Part model, mm, in its own coordinate system. A direction names the side the tool comes from. Coordinates: 2 decimals unless noted, no trailing zeros. Order: outer loops, then holes, each group sorted by start corner. A loop starts at its lowest first (then second) coordinate and runs counter-clockwise, first axis right, second up. Notation, with made-up numbers: M 9,82 L 68,82 A11 ccw 68,101 Z; hole C 61.25,-25 d6. An arc over 180 degrees is marked long. Answer in a Markdown table with one row per item. Add a question column.
from build123d import *

# Parameters (mm, degrees)
BOSS_EXTRUDE1_DEPTH = 10
BOSS_EXTRUDE2_DEPTH = 8
SKETCH4_R           = 13
CUT_EXTRUDE2_DEPTH  = 77.40353395
SKETCH5_W           = 4
SKETCH5_H           = 38
SKETCH5_R           = 1
BOSS_EXTRUDE3_DEPTH = 10


with BuildPart() as part:
    # Sketch1 → Boss-Extrude1 (new body)
    with BuildSketch(Plane(origin=(0, 0, 0), x_dir=(0, 1, 0), z_dir=(0, 0, 1))):
        with BuildLine():
            Line((-25, -37.5), (25, -37.5))
            ThreePointArc((25, -37.5), (33.838834765, -33.838834765), (37.5, -25))
            Line((37.5, -25), (37.5, 25))
            ThreePointArc((37.5, 25), (33.838834765, 33.838834765), (25, 37.5))
            Line((25, 37.5), (-25, 37.5))
            ThreePointArc((-25, 37.5), (-33.838834765, 33.838834765), (-37.5, 25))
            Line((-37.5, 25), (-37.5, -25))
            ThreePointArc((-37.5, -25), (-33.838834765, -33.838834765), (-25, -37.5))
        make_face()
    extrude(amount=BOSS_EXTRUDE1_DEPTH)

    # Sketch2 → Boss-Extrude2 (add)
    with BuildSketch(Plane.YZ.offset(37.5)):
        with BuildLine():
            ThreePointArc((14.587782351, 53.492363969), (0, 65), (-14.587782351, 53.492363969))
            Line((-14.587782351, 53.492363969), (-25, 10))
            Line((-25, 10), (25, 10))
            Line((25, 10), (14.587782351, 53.492363969))
        make_face()
        with BuildLine():
            ThreePointArc((0, 44), (-5.795554958, 48.447085729), (-3, 55.196152423))
            Line((-3, 55.196152423), (3, 55.196152423))
            ThreePointArc((3, 55.196152423), (5.795554958, 48.447085729), (0, 44))
        make_face(mode=Mode.SUBTRACT)
    boss_extrude2 = extrude(amount=-BOSS_EXTRUDE2_DEPTH)

    # Mirror1: Boss-Extrude2 across plane
    add(boss_extrude2.mirror(Plane(origin=(0, 0, 0), x_dir=(0, 0, 1), z_dir=(1, 0, 0))))

    # Sketch4 → Cut-Extrude2 (cut, through all)
    with BuildSketch(Plane.XY.offset(10)):
        Circle(SKETCH4_R)
    extrude(amount=-CUT_EXTRUDE2_DEPTH, mode=Mode.SUBTRACT)

    # Sketch5 → Boss-Extrude3 (add)
    # profile 1 of 2: a face of its own
    with BuildSketch(Plane.XY.offset(10)):
        with Locations((-15, 12.5)):
            Rectangle(SKETCH5_W, SKETCH5_H)
        with Locations((-15, -4.5)):
            Circle(SKETCH5_R, mode=Mode.SUBTRACT)
        with Locations((-15, 29.5)):
            Circle(SKETCH5_R, mode=Mode.SUBTRACT)
    # profile 2 of 2: a face of its own
    with BuildSketch(Plane.XY.offset(10)):
        with Locations((15, 12.5)):
            Rectangle(SKETCH5_W, SKETCH5_H)
        with Locations((15, -4.5)):
            Circle(SKETCH5_R, mode=Mode.SUBTRACT)
        with Locations((15, 29.5)):
            Circle(SKETCH5_R, mode=Mode.SUBTRACT)
    extrude(amount=BOSS_EXTRUDE3_DEPTH)


solid = part.part
(1) Drop flat-ended pins along their axis: P1, Ø1.6, axis at x = 15, y = 29.5, coming from the +Z side; P2, Ø4.5, axis at x = -16, z = 16.5, coming from the -Y side; P3, Ø2, axis at x = -15.5, z = 16.5, coming from the +Y side. Give the stop position or say it passes through.
(2) Slice it at D-D (y = -21.5). List the corners of the cut face in (x, z).
(3) 3-axis set-ups, long thin cutter, end or side, ignore diameter. For faces 4 (the cylindrical face through (-10.316, -7.91, 5.07)), 5 (the flat face through (-15, -6.5, 15)), 6 (the cylindrical face through (15.54, 30.34, 14.93)), 7 (the flat face through (15, 31.5, 15)), 8 (the flat face through (13, 12, 15)): which of +Z, -Z, +X, -X, +Y, -Y reach the whole face in a straight line?
(4) Pull direction Y, two halves, no side cores. Call faces 1 (the cylindrical face through (-33.935, -33.741, 4.93)), 2 (the cylindrical face through (-34, 0, 65)), 3 (the flat face through (-15, -5, 10)): pulls with the +Y half, pulls with the -Y half, needs draft (parallel to the pull), parting line crosses it, or undercut.
(5) Slice it at A-A (x = 12). List the corners of the cut face in (y, z).
(6) Wall check: line 1 (Y direction, x = -15, z = 13); line 2 (X direction, y = -11, z = 10.5); line 3 (X direction, y = -4, z = 15). Give the ranges that are in metal, low to high.
(7) Slice it at C-C (z = 39.5). List the corners of the cut face in (x, y).
(8) Slice it at B-B (x = -15). List the corners of the cut face in (y, z), and give its area (3 significant figures).
Computed:
| question | item | result |
|---|---|---|
| 1 | P1 | stops at z = 10 |
| 1 | P2 | stops at y = -6.5 |
| 1 | P3 | stops at y = 31.5 |
| 2 | outline | M -37.5,0 L 37.5,0 L 37.5,24.62 L 29.5,24.62 L 29.5,10 L -29.5,10 L -29.5,24.62 L -37.5,24.62 Z |
| 3 | face 4 | +Z, -Z |
| 3 | face 5 | +Z, -Y |
| 3 | face 6 | +Z |
| 3 | face 7 | +Z, +X, -X, +Y |
| 3 | face 8 | +Z, +Y, -Y |
| 4 | face 1 | pulls with the -Y half |
| 4 | face 2 | parting line crosses it |
| 4 | face 3 | undercut |
| 5 | outline | M -37.5,0 L -5,0 L -5,10 L -37.5,10 Z; M 5,0 L 37.5,0 L 37.5,10 L 5,10 Z |
| 6 | line 1 | y = -6.5 to -5.5, -3.5 to 28.5, 30.5 to 31.5 |
| 6 | line 2 | x = -37.5 to -29.5, 29.5 to 37.5 |
| 6 | line 3 | x = -37.5 to -29.5, -17 to -15.87, -14.13 to -13, 13 to 14.13, 15.87 to 17, 29.5 to 37.5 |
| 7 | outline | M -37.5,-17.94 L -29.5,-17.94 L -29.5,17.94 L -37.5,17.94 Z; M 29.5,-17.94 L 37.5,-17.94 L 37.5,17.94 L 29.5,17.94 Z |
| 8 | outline | M -37.5,0 L 37.5,0 L 37.5,10 L 31.5,10 L 31.5,20 L 30.5,20 L 30.5,10 L 28.5,10 L 28.5,20 L -3.5,20 L -3.5,10 L -5.5,10 L -5.5,20 L -6.5,20 L -6.5,10 L -37.5,10 Z |
| 8 | area | 1,090 mm^2 |
